```python
from build123d import *

# Parameters (mm, degrees)
SKETCH1_W           = 19.65
SKETCH1_H           = 6
BOSS_EXTRUDE1_DEPTH = 10.16
SKETCH2_R           = 0.25
BOSS_EXTRUDE2_DEPTH = 4.1


with BuildPart() as part:
    # Sketch1 → Boss-Extrude1 (new body)
    with BuildSketch(Plane(origin=(0, 0, 0), x_dir=(1, 0, 0), z_dir=(0, 1, 0))):
        Rectangle(SKETCH1_W, SKETCH1_H)
    extrude(amount=BOSS_EXTRUDE1_DEPTH)

    # Sketch2 → Boss-Extrude2 (add)
    with BuildSketch(Plane.XZ):
        with Locations(Location((0.005, -2.1, 0), (0, 0, 90))):
            Circle(SKETCH2_R)
        with Locations(Location((2.545, -2.1, 0), (0, 0, 90))):
            Circle(SKETCH2_R)
        with Locations(Location((5.085, -2.1, 0), (0, 0, 90))):
            Circle(SKETCH2_R)
        with Locations(Location((-5.075, -2.1, 0), (0, 0, 90))):
            Circle(SKETCH2_R)
        with Locations(Location((-7.615, -2.1, 0), (0, 0, 90))):
            Circle(SKETCH2_R)
    extrude(amount=BOSS_EXTRUDE2_DEPTH)


solid = part.part
```
Geometry check sheet. Reference: the model listing, model coordinates, mm. Round coordinates to 2 decimals unless told otherwise and drop trailing zeros. Order: outer loops, then holes, each group sorted by start corner. A loop starts at its lowest first (then second) coordinate and runs counter-clockwise, first axis right, second up. Notation, with made-up numbers: (25, -21) -> (50, -21) arc R33 ccw to (50, 13) -> close; hole circle Ø2 at (63, 43). An arc over 180 degrees is marked (long way). Return JSON: item names as keys, results as strings. Group by question number.
Q1. Section check B-B, the plane y = -2.75. Record the boundary of the cut face in (x, z) (3 decimals).
Q2. Release check for a two-part mould opening along Z. For faces 1 (the flat face through (0, 0, 0)), 2 (the flat face through (0, 5, 3)), 3 (the flat face through (0, 5, -3)) record: released by +Z, released by -Z, zero draft, split by the parting line, or undercut.
Q3. Material ranges on probe 1 along Y at (x, z) = (-8, 1.4), recorded low to high. Write a range as from..to.
Q4. Gauge pin test, flat ends, axial feed: pin 1 (1 mm diameter, centred on x = 5, z = 0.5, fed in from -Y); pin 2 (1.5 mm diameter, centred on x = 2.5, z = -1.5, fed in from -Y). Record the tip position at first contact, or that the pin passes through.
Q5. Section check C-C, the plane x = -4.5. Record the boundary of the cut face in (y, z).
Q6. Section check A-A, the plane z = -2.1. Record the boundary of the cut face in (x, y) (3 decimals), plus the area to 3 significant figures.
Numbers:
{
 "1": {"outline": "circle Ø0.5 at (-7.615, -2.1); circle Ø0.5 at (-5.075, -2.1); circle Ø0.5 at (0.005, -2.1); circle Ø0.5 at (2.545, -2.1); circle Ø0.5 at (5.085, -2.1)"},
 "2": {"face 1": "zero draft", "face 2": "released by +Z", "face 3": "released by -Z"},
 "3": {"probe 1": "0..10.16"},
 "4": {"pin 1": "y = 0", "pin 2": "y = -4.1"},
 "5": {"outline": "(0, -3) -> (10.16, -3) -> (10.16, 3) -> (0, 3) -> close"},
 "6": {"outline": "(-9.825, 0) -> (-7.865, 0) -> (-7.865, -4.1) -> (-7.365, -4.1) -> (-7.365, 0) -> (-5.325, 0) -> (-5.325, -4.1) -> (-4.825, -4.1) -> (-4.825, 0) -> (-0.245, 0) -> (-0.245, -4.1) -> (0.255, -4.1) -> (0.255, 0) -> (2.295, 0) -> (2.295, -4.1) -> (2.795, -4.1) -> (2.795, 0) -> (4.835, 0) -> (4.835, -4.1) -> (5.335, -4.1) -> (5.335, 0) -> (9.825, 0) -> (9.825, 10.16) -> (-9.825, 10.16) -> close", "area": "210 mm^2"}
}
